```python
from build123d import *

# Parameters (mm, degrees)
BASEHEAD_DEPTH = 6.63
SKETCH4_W      = 0.6
SKETCH4_H      = 11.237604307


# Read off the part's stored shape, not the designer's step: HeadChamfer
with BuildPart() as part:
    # Sketch1 → BaseHead (new body)
    with BuildSketch(Plane(origin=(0, 0, 0), x_dir=(0, 0, -1), z_dir=(1, 0, 0))):
        Polygon((8, 4.618802154), (8, -4.618802154), (0, -9.237604307), (-8, -4.618802154), (-8, 4.618802154), (0, 9.237604307), align=None)
    extrude(amount=BASEHEAD_DEPTH)

    # HeadChamfer outline → HeadChamfer (revolve, cut)
    with BuildSketch(Plane.YX):
        Polygon((9.237604311, 0.714531182), (8, 0), (9.237604311, 0), align=None)
    revolve(axis=Axis((0, 0, 0), (1, 0, 0)), mode=Mode.SUBTRACT)

    # HeadChamfer 2 outline → HeadChamfer 2 (revolve)
    with BuildSketch(Plane.YX):
        Polygon((5, 6.63), (5, 45.802), (4.172, 46.63), (0, 46.63), (0, 6.63), align=None)
    revolve(axis=Axis((0, 0, 0), (1, 0, 0)))

    # Sketch4 → BearingFace (revolve, cut)
    with BuildSketch(Plane.XY, mode=Mode.PRIVATE) as bearingface_sk:
        with Locations((6.33, 13.618802154)):
            Rectangle(SKETCH4_W, SKETCH4_H)
    revolve(bearingface_sk.sketch.rotate(Axis((0, 0, 0), (1, 0, 0)), 90), axis=Axis((0, 0, 0), (1, 0, 0)), mode=Mode.SUBTRACT)


solid = part.part
```
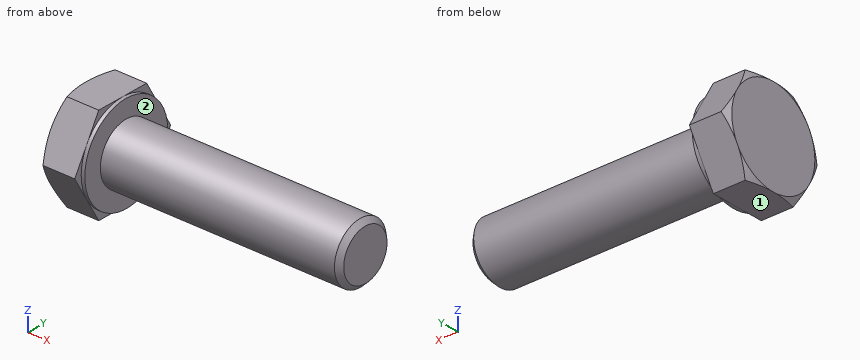
Can you work these out from the model? Positions are in its coordinate system, mm. Face numbers are marked on the shaded views. A direction names the side the tool comes from. Give positions to 0.01 mm unless a question says otherwise; leave off trailing zeros. Write each loop counter-clockwise with the first axis right and the second up, starting at its lowest first coordinate (ties: lowest second). Pieces come first, ordered by that corner, then holes. Notation, with made-up numbers: (24.25, 62.25) -> (50.25, 62.25) arc R8 cw to (50.25, 76.25) -> close; hole circle Ø1 at (62, -37.75). An arc over 180 degrees is marked (long way). Write item = value, one per line.
(1) For the marked faces 1 and 2, which set-ups out of +Z, -Z, +X, -X, +Y, -Y let a thin tool reach every point of the face, with its end or its side?
Worked out:
face_1 = -Z, +X, -X, +Y, -Y
face_2 = +X
(2) Suppose I cut it at A-A on x = 3. Write out the boundary of the cut face in (y, z), then the cut area to 3 significant figures.
Worked out:
outline = (-9.24, 0) -> (-4.62, -8) -> (4.62, -8) -> (9.24, 0) -> (4.62, 8) -> (-4.62, 8) -> close
area = 222 mm^2
(3) Suppose I cut it at B-B on x = 11. Write out the boundary of the cut face in (y, z), then the cut area to 3 significant figures.
Worked out:
outline = circle Ø10 at (0, 0)
area = 78.5 mm^2
(4) I'm going to push flat-ended pins straight in: P1, Ø1.2, axis at y = -5, z = 6, coming from the +X side; P2, Ø3, axis at y = -4, z = -5, coming from the +X side; P3, Ø6, axis at x = 13, y = 4, coming from the +Z side. Where does each tip first touch, or does it pass through?
Worked out:
P1 = 6.63
P2 = 45.9
P3 = 4.9
(5) I need wall thicknesses on probe 1 along Z at (x, y) = (9.5, 0.25); probe 2 along X at (y, z) = (-2, 4.75); probe 3 along Y at (x, z) = (22, -3). Which ranges of each line are inside material? Lowest first, please. Write a range as from..to.
Worked out:
probe_1 = -4.99..4.99
probe_2 = 0..6.63
probe_3 = -4..4
